Could you check a few things on this drawing? It's one solid part, dimensions in mm from its lowest x, y, z. A direction names the side the tool comes from. Give positions to 0.01 mm unless a question says otherwise; leave off trailing zeros. Loops run counter-clockwise (first coordinate to the right, second up) from the corner with the lowest first, then second, coordinate; pieces in that order, holes last. Notation, with made-up numbers: (-1, 24) -> (33, 24) arc R16 ccw to (33, 29) -> close; hole circle Ø3 at (51.25, 7.5). An arc over 180 degrees is marked (long way). One line per question, with ' | ' between items.
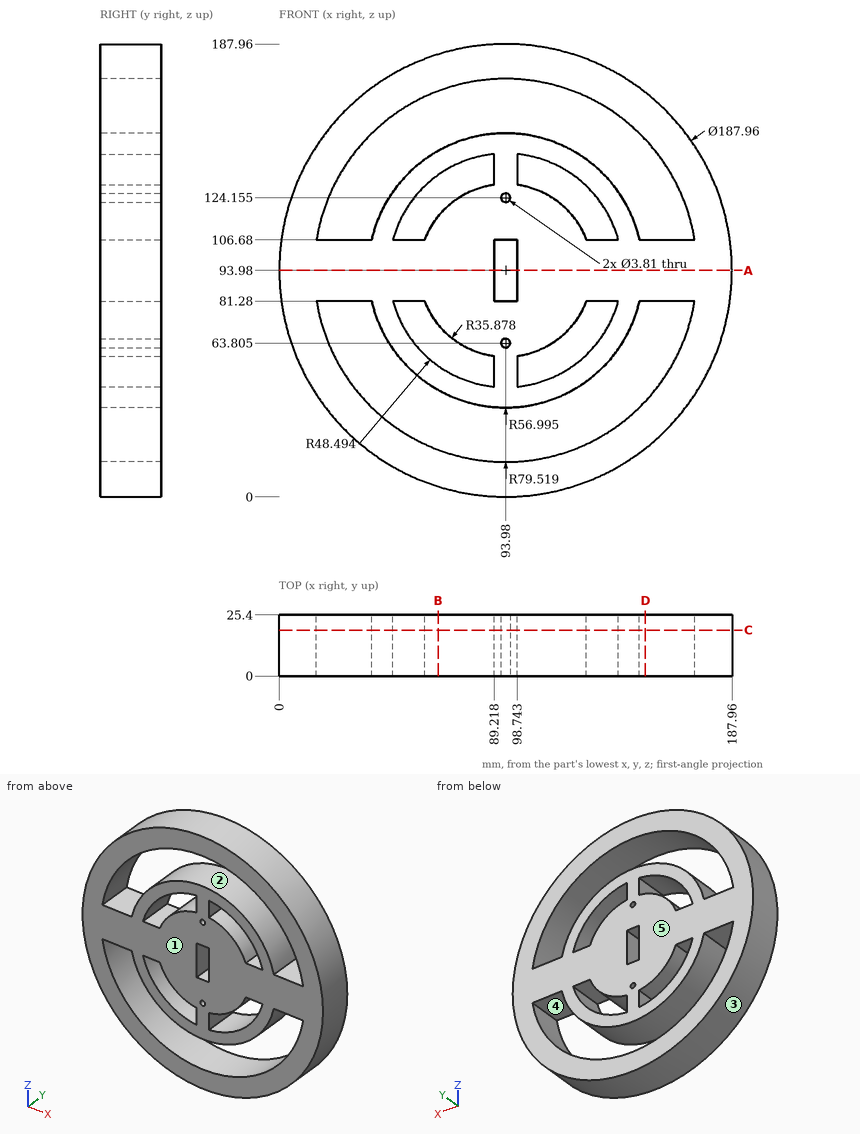
Q1. If we section it at D-D (x = 152): Write out the boundary of the cut face in (y, z).
Entries:
outline: (0, 20.05) -> (25.4, 20.05) -> (25.4, 39.6) -> (0, 39.6) -> close; (0, 81.28) -> (25.4, 81.28) -> (25.4, 106.68) -> (0, 106.68) -> close; (0, 148.36) -> (25.4, 148.36) -> (25.4, 167.91) -> (0, 167.91) -> close
Q2. If we section it at A-A (z = 93.98): Write out the boundary of the cut face in (x, y), plus the area to 3 significant figures.
Entries:
outline: (0, 0) -> (89.22, 0) -> (89.22, 25.4) -> (0, 25.4) -> close; (98.74, 0) -> (187.96, 0) -> (187.96, 25.4) -> (98.74, 25.4) -> close | area: 4,530 mm²
Q3. If we section it at B-B (x = 66): Write out the boundary of the cut face in (y, z) (1 decimal).
Entries:
outline: (0, 4.3) -> (25.4, 4.3) -> (25.4, 19.5) -> (0, 19.5) -> close; (0, 44.3) -> (25.4, 44.3) -> (25.4, 54.4) -> (0, 54.4) -> close; (0, 71.5) -> (25.4, 71.5) -> (25.4, 116.4) -> (0, 116.4) -> close; (0, 133.6) -> (25.4, 133.6) -> (25.4, 143.6) -> (0, 143.6) -> close; (0, 168.4) -> (25.4, 168.4) -> (25.4, 183.7) -> (0, 183.7) -> close
Q4. For pin 1 Ø3 at (x, y) = (101.5, 5) entering from +Z; pin 2 Ø14.5 at (x, y) = (54.5, 10.5) entering from -Z; pin 3 Ø10 at (x, z) = (116, 27) entering from -Y (3 decimals); pin 4 Ø10 at (y, z) = (17.5, 134) entering from +X, each with a flat end and sliding along its axis, tell me the tip position at first contact or that it passes through.
Entries:
pin 1: z = 187.77 | pin 2: z = 5.7 | pin 3: through | pin 4: x = 181.19
Q5. On a 3-axis mill with a long thin cutter (end or side, diameter ignored), from which of +Z, -Z, +X, -X, +Y, -Y can I reach the whole of each face in a straight line? I mean the marked faces 4 and 5. Say none if no direction works.
Entries:
face 4: +Y, -Y | face 5: +Z, -Z, +X, -X, +Y
Q6. If we mould it in two halves opening along Z, with no side actions, what happens to the marked faces 1, 2 and 3? For each: pulls with the +Z half, pulls with the -Z half, needs draft (parallel to the pull), parting line crosses it, or undercut.
Entries:
face 1: needs draft | face 2: undercut | face 3: parting line crosses it
Q7. If we section it at C-C (y = 19): State how many separate pieces and enclosed holes the cut face has, plus the area to 3 significant figures.
Entries:
separate pieces: 1 | enclosed holes: 9 | area: 16,500 mm²
Q8. If I drill on probe 1 along X at (y, z) = (19.75, 117) (1 decimal); probe 2 along Z at (x, y) = (90.5, 22.25) (1 decimal); probe 3 along X at (y, z) = (24.5, 79) (1 decimal), over which ranges is the centre line in solid material (lowest first)? Write a range as from..to.
Entries:
probe 1: 2.9..17.9, 41.8..51.3, 66.5..121.5, 136.7..146.1, 170.1..185.1 | probe 2: 0.1..14.5, 37.1..81.3, 106.7..150.9, 173.4..187.9 | probe 3: 1.2..15.9, 39..47.9, 61.4..126.6, 140.1..149, 172.1..186.8
